Autodesk Inventor part; units mm, degrees
ref_plane "YZ Plane" through (0, 0, 0) normal (1, 0, 0) x (0, 1, 0)
ref_plane "XZ Plane" through (0, 0, 0) normal (0, 1, 0) x (-1, 0, 0)
ref_plane "XY Plane" through (0, 0, 0) normal (0, 0, 1) x (1, 0, 0)
sketch "Эскиз1" plane through (0, 0, 0) normal (0, 0, 1) x (1, 0, 0)
  line L0 (0, 0) -> (190, 0)
  line L1 (190, 0) -> (190, 640)
  line L2 (190, 640) -> (215, 640)
  line L3 (215, 640) -> (215, 630)
  line L4 (215, 630) -> (200, 630)
  line L5 (200, 630) -> (200, 0)
  line L6 (200, 0) -> (190, 0)
  line L7 (0, -128) -> (0, 768)
  line L8 (200, 0) -> (200, 2)
  line L9 (200, 2) -> (190, 2)
  dimension "d0" = 190
  dimension "d1" = 640
  dimension "d2" = 25
  dimension "d3" = 10
  dimension "d20" = 2
revolve "Вращение1" add sketch "Эскиз1" angle 360 about axis through (0, -10, 0) along (0, 1, 0) contours L1 L2 L3 L4 L5 L9
sketch "Эскиз2" plane through (0, 640, 0) normal (0, 1, 0) x (1, 0, 0)
  circle A0 centre (207, 0) radius 4
  circle A1 centre (0, 0) radius 190
  line L0 (190, 0) -> (207, 0)
  dimension "d6" = 8
  dimension "d19" = 17
extrude "Выдавливание1" cut sketch "Эскиз2" against normal through all contours A0
sketch "Эскиз3" plane through (0, 0, 0) normal (1, 0, 0) x (0, 1, 0)
  line L0 (630, 215) -> (630, -215)
  line L1 (630, 200) -> (630, -200)
  line L2 (630, 0) -> (529, 0)
  circle A0 centre (529, 0) radius 50
  line L3 (0, 0) -> (0, 0)
  circle A1 centre (0, 0) radius 50
  dimension "d11" = 101
  dimension "d12" = 100
  dimension "d17" = 0
  dimension "d18" = 100
extrude "Выдавливание2" cut sketch "Эскиз3" along normal through all both and the other way through all
properties part number "Втулка_CPY" material "Сталь, легированная"
Verification items for the finished model (mm, model axes). A direction names the side the tool comes from. Coordinates: 2 decimals unless noted, no trailing zeros. Order: outer loops, then holes, each group sorted by start corner. A loop starts at its lowest first (then second) coordinate and runs counter-clockwise, first axis right, second up.
1. Release check for a two-part mould opening along Z. For faces 3 (the face through (-170.62, 634.93, -130.82)), 4 (the face through (-191.54, 49.99, -1.07)), 5 (the face through (-1, 2, 191)) record: +Z half, -Z half, draft (parallel to the pull), parting line (faces both ways), or undercut.
Results found:
face 3: parting line
face 4: undercut
face 5: draft
2. Go/stop test with flat-tipped pins: pin 1 Ø6.5 at (x, z) = (207, 0) entering from +Y; pin 2 Ø1 at (y, z) = (187, 23.5) entering from -X; pin 3 Ø5 at (x, y) = (10.5, 296) entering from -Z; pin 4 Ø3 at (x, y) = (78.5, 542.5) entering from -Z. Record where each tip stops, or that it passes through.
Results found:
pin 1: passes through
pin 2: stops at x = -198.67
pin 3: stops at z = -199.84
pin 4: stops at z = -184.58
3. Sectioned sample at C-C, the plane z = 84. Record the cut outline in (x, y), and give its area (3 significant figures).
Results found:
outline: (-197.91, 630) - (-181.5, 630) - (-181.5, 2) - (-170.42, 2) - (-170.42, 640) - (-197.91, 640) - close; (170.42, 2) - (181.5, 2) - (181.5, 630) - (197.91, 630) - (197.91, 640) - (170.42, 640) - close
area: 14,500 mm2
4. Set-up check for faces 1 (the face through (190.764, 311.604, 60.075)), 2 (the face through (181.226, 325.466, -57.071)): record each of +Z, -Z, +X, -X, +Y, -Y from which the full face is reachable in a straight line by a thin tool's end or side.
Results found:
face 1: -Y
face 2: +Y, -Y
5. Scan lines: line 1 (Y direction, x = -191.5, z = 0); line 2 (X direction, y = 474, z = 10); line 3 (X direction, y = 609, z = 18.5). Record each from-to range of solid material in increasing order.
Results found:
line 1: y = 50 to 479, 579 to 640
line 2: x = -199.75 to -189.74, 189.74 to 199.75
line 3: x = -199.14 to -189.1, 189.1 to 199.14
6. Sectioned sample at D-D, the plane z = -30.5. Record the cut outline in (x, y).
Results found:
outline: (-212.83, 630) - (-197.66, 630) - (-197.66, 568.62) - (-187.54, 568.62) - (-187.54, 640) - (-212.83, 640) - close; (-197.66, 39.62) - (-187.54, 39.62) - (-187.54, 489.38) - (-197.66, 489.38) - close; (187.54, 39.62) - (197.66, 39.62) - (197.66, 489.38) - (187.54, 489.38) - close; (187.54, 568.62) - (197.66, 568.62) - (197.66, 630) - (212.83, 630) - (212.83, 640) - (187.54, 640) - close
7. Sectioned sample at A-A, the plane x = 0. Record the cut outline in (y, z), and give its area (3 significant figures).
Results found:
outline: (2, -200) - (630, -200) - (630, -215) - (640, -215) - (640, -190) - (2, -190) - close; (2, 190) - (640, 190) - (640, 215) - (630, 215) - (630, 200) - (2, 200) - close
area: 13,100 mm2
8. Sectioned sample at B-B, the plane y = 493. Record the cut outline in (x, z), and give its area (3 significant figures).
Results found:
outline: (-196.97, -34.7) arc R200 ccw to (196.97, -34.7) - (186.8, -34.7) arc R190 cw to (-186.8, -34.7) - close; (-196.97, 34.7) - (-186.8, 34.7) arc R190 cw to (186.8, 34.7) - (196.97, 34.7) arc R200 ccw to start
area: 10,900 mm2
